Autodesk Inventor part; units mm, degrees
ref_plane "工作平面1" through (0, -17.5, 0) normal (0, 1, 0) x (1, 0, 0)
ref_plane "YZ Plane" through (0, 0, 0) normal (1, 0, 0) x (0, 1, 0)
ref_plane "XZ Plane" through (0, 0, 0) normal (0, 1, 0) x (-1, 0, 0)
sketch "草圖1" plane through (0, 0, 0) normal (0, 1, 0) x (-1, 0, 0)
  line L0 (22.9, 7.0791) -> (-22.9, 7.0791)
  line L1 (-22.9, 7.0791) -> (-22.9, -19.9209)
  line L2 (-20.9, -21.9209) -> (20.9, -21.9209)
  line L3 (22.9, -19.9209) -> (22.9, 7.0791)
  arc A0 (20.9, -21.9209) -> (22.9, -19.9209) centre (20.9, -19.9209) ccw
  arc A1 (-22.9, -19.9209) -> (-20.9, -21.9209) centre (-20.9, -19.9209) ccw
  line L4 (0, -28.2179) -> (0, 12.962)
  circle A2 centre (0, -16.9209) radius 2
  circle A3 centre (-18, -16.9209) radius 2
  circle A4 centre (18, -16.9209) radius 2
  point P0 (0, 0)
  dimension "d2" = 2
  dimension "d3" = 4
  dimension "d4" = 18
  dimension "d5" = 4
  dimension "d6" = 24
  dimension "d9" = 5
extrude "擠出1" add sketch "草圖1" along normal mid plane 5 contours L3 A0 L2 L4 A2 L0 | L4 A2 L2 A1 L1 L0
sketch "草圖3" plane through (-22.9, 2.5, 7.0791) normal (0, 0, 1) x (1, 0, 0)
  line L0 (0, -5) -> (0, 0)
  line L1 (0, 0) -> (45.8, 0)
  line L2 (45.8, -5) -> (45.8, 0)
  line L3 (0, 0) -> (45.8, 0)
  line L4 (45.8, 0) -> (45.8, -5)
  line L5 (0, -5) -> (0, 0)
  line L6 (0, 0) -> (45.8, -5) construction
  line L7 (45.8, 0) -> (0, -5) construction
  line L8 (24.9, -5) -> (20.9, -5)
  line L9 (-18.1, -5) -> (63.9, -5)
  line L10 (-18.1, -5) -> (-18.1, -28)
  line L11 (-18.1, -28) -> (63.9, -28)
  line L12 (63.9, -28) -> (63.9, -5)
  point P0 (22.9, -2.5)
  point P1 (22.9, -5)
  dimension "d12" = 82
  dimension "d13" = 23
extrude "擠出2" add sketch "草圖3" along normal blind 10
ref_plane "工作平面1" through (0, -17.5, 0) normal (0, 1, 0) x (1, 0, 0)
sketch "草圖5" plane through (0, -17.5, 0) normal (0, 1, 0) x (1, 0, 0)
  line L0 (-41, -17.0791) -> (41, -17.0791)
  line L1 (-41, -17.0791) -> (41, -17.0791)
  line L2 (41, -17.0791) -> (41, -62.0791)
  line L3 (0, -103.0791) -> (0, -103.0791)
  line L4 (-41, -62.0791) -> (-41, -17.0791)
  arc A0 (0, -103.0791) -> (41, -62.0791) centre (0, -62.0791) ccw
  arc A1 (-41, -62.0791) -> (0, -103.0791) centre (0, -62.0791) ccw
  point P0 (0, 0)
  point P1 (41, -103.0791)
  point P2 (-41, -103.0791)
  point P3 (41, -17.0791)
  point P4 (0, -103.0791)
  dimension "d19" = 86
  dimension "d22" = 41
  dimension "d23" = 41
  dimension "d37" = 82
extrude "擠出3" add sketch "草圖5" against normal up to surface (8 mm away)
sketch "草圖6" plane through (0, -17.5, 0) normal (0, 1, 0) x (1, 0, 0)
  arc A0 (-41, -62.0791) -> (41, -62.0791) centre (0, -62.0791) ccw
  circle A1 centre (0, -60.0791) radius 38.5
  line L0 (-41, -17.0791) -> (41, -17.0791)
  point P0 (0, 0)
  dimension "d24" = 77
  dimension "d28" = 43
fillet "圓角2" radius 2 1 edges at (0, -17.5, 17.0791)
extrude "擠出5" cut sketch "草圖6" against normal blind 1
sketch "草圖8" plane through (0, -18.5, 60.0791) normal (0, 1, 0) x (1, 0, 0)
  circle A0 centre (-20.8595, 21.4584) radius 1.6
  circle A1 centre (0, 0) radius 38.5
  line L0 (0, 107) -> (0, -68)
  circle A2 centre (20.8595, 21.4584) radius 1.6
  circle A3 centre (20.8595, -20.2606) radius 1.6
  circle A4 centre (-20.8595, -20.2606) radius 1.6
  point P0 (0, 60.0791)
  dimension "d32" = 3.2
  dimension "d33" = 41.719
  dimension "d38" = 41.719
extrude "擠出6" cut sketch "草圖8" against normal through all contours A0 | A2 | A3 | A4
fillet "圓角3" radius 2 3 edges at (22.9, -2.5, 12.0791) (-22.9, -2.5, 12.0791) (0, -2.5, 7.0791)
sketch "草圖9" plane through (41, -25.5, 7.0791) normal (1, 0, 0) x (0, 0, -1)
  line L0 (-55, 0) -> (-96, 0)
  line L1 (0, 23) -> (0, 0)
  line L2 (-96, 0) -> (0, 0)
  line L3 (0, 0) -> (0, 2)
  line L4 (0, 2) -> (-96, 2)
  line L5 (-96, 2) -> (-96, 0)
  point P0 (7.0791, 25.5)
  dimension "d39" = 2
extrude "擠出7" cut sketch "草圖9" against normal through all
properties part number "lidar base"
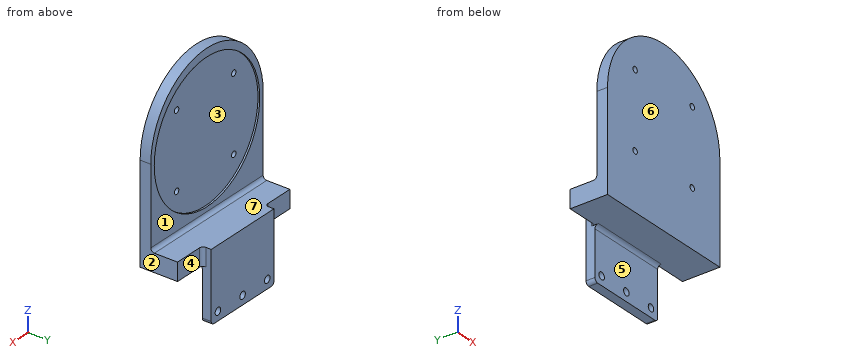
Geometry check sheet. Reference: the model listing, model coordinates, mm. Face numbers are marked on the shaded views. A direction names the side the tool comes from. Give positions to 0.01 mm unless a question says otherwise; leave off trailing zeros. Loops run counter-clockwise (first coordinate to the right, second up) from the corner with the lowest first, then second, coordinate; pieces in that order, holes last.
(1) Set-up check for the marked faces 4, 5, 6 and 7: record each of +Z, -Z, +X, -X, +Y, -Y from which the full face is reachable in a straight line by a thin tool's end or side.
From the geometry:
face 4: +Z, -Z, +X, +Y
face 5: -Z, +X, -X, -Y
face 6: +Z, -Z, +X, -X, -Y
face 7: +Z, +X, -X, +Y
(2) Depth check by flat-ended pin: pin 1 Ø6.5 at (x, z) = (0, -16.92) entering from -Y; pin 2 Ø5 at (x, y) = (-11, -7.5) entering from -Z; pin 3 Ø3.5 at (y, z) = (0, -9.5) entering from -X; pin 4 Ø12 at (y, z) = (-19, 67) entering from -X. Enter the tip coordinate at first touch or a pass-through.
From the geometry:
pin 1: stops at y = -2.5
pin 2: stops at z = 7.08
pin 3: stops at x = -22.9
pin 4: stops at x = -41
(3) Section check C-C on x = 14. Record the cut outline in (y, z), then the cut area to 3 significant figures.
From the geometry:
outline: (-23.5, 7.08) - (-4.5, 7.08) arc R2 cw to (-2.5, 5.08) - (-2.5, -21.92) - (2.5, -21.92) - (2.5, 17.08) - (-15.5, 17.08) arc R2 cw to (-17.5, 19.08) - (-17.5, 24.21) - (-18.5, 24.21) - (-18.5, 95.94) - (-17.5, 95.94) - (-17.5, 100.61) - (-23.5, 100.61) - close
area: 836 mm2
(4) Section check A-A on x = 0. Record the cut outline in (y, z).
From the geometry:
outline: (-23.5, 7.08) - (-4.5, 7.08) arc R2 cw to (-2.5, 5.08) - (-2.5, -14.92) - (2.5, -14.92) - (2.5, 17.08) - (-15.5, 17.08) arc R2 cw to (-17.5, 19.08) - (-17.5, 21.58) - (-18.5, 21.58) - (-18.5, 98.58) - (-17.5, 98.58) - (-17.5, 103.08) - (-23.5, 103.08) - close; (-2.5, -21.92) - (2.5, -21.92) - (2.5, -18.92) - (-2.5, -18.92) - close
(5) Section check D-D on y = -13.75. Record the cut outline in (x, z).
From the geometry:
outline: (-41, 7.08) - (41, 7.08) - (41, 17.08) - (-41, 17.08) - close
(6) Release check for a two-part mould opening along X. For the marked faces 1, 2 and 3 record: released by +X, released by -X, zero draft, split by the parting line, or undercut.
From the geometry:
face 1: zero draft
face 2: released by +X
face 3: undercut
(7) Thickness scan on L1, parallel to Z at x = 0, y = -1.5; L2, parallel to Y at x = 21, z = 56; L3, parallel to Y at x = -0.5, z = 21. Record the ranges inside material, lowest first.
From the geometry:
L1: z = -21.92 to -18.92, -14.92 to 17.08
L2: y = -23.5 to -18.5
L3: y = -23.5 to -17.5
(8) Section check B-B on z = 8.5. Record the cut outline in (x, y).
From the geometry:
outline: (-41, -23.5) - (41, -23.5) - (41, -2.5) - (24.9, -2.5) arc R2 cw to (22.9, -0.5) - (22.9, 2.5) - (-22.9, 2.5) - (-22.9, -0.5) arc R2 cw to (-24.9, -2.5) - (-41, -2.5) - close
